Part model, mm, in its own coordinate system. Round coordinates to 2 decimals unless told otherwise and drop trailing zeros. Write each loop counter-clockwise with the first axis right and the second up, starting at its lowest first coordinate (ties: lowest second). Pieces come first, ordered by that corner, then holes. Notation, with made-up numbers: M 27.25,53.25 L 39.25,53.25 A18 ccw 39.25,87.25 Z; hole C 37,12.5 d3. An arc over 180 degrees is marked long. Use a Markdown table: item, result. Add a question column.
1) Drop flat-ended pins along their axis: P1, Ø10, axis at y = -9, z = 11, coming from the -X side; P2, Ø6, axis at y = -4.5, z = -7.5, coming from the +X side; P3, Ø10, axis at x = 7, y = -4, coming from the -Z side. Give the stop position or say it passes through.
2) Slice it at C-C on z = -9. Write the cut outline in (x, y).
3) Wall check: probe 1 along X at (y, z) = (-14.5, 0); probe 2 along Z at (x, y) = (9, -10.5); probe 3 along X at (y, z) = (-6, -4.5). Give the ranges that are in metal, low to high.
4) Slice it at B-B on z = -3. Write the cut outline in (x, y).
5) Slice it at A-A on x = 0. Write the cut outline in (y, z), plus the area to 3 significant figures.
6) Two-plate mould, pull along X, no slides. Class faces 1 (the face through (12.626, -10.018, 12.518)), 2 (the face through (-12.518, -10.018, 12.626)), 3 (the face through (-5.299, -10.018, -12.926)), 4 (the face through (-5.056, -10.018, 16.036)): released by +X, released by -X, zero draft, split by the parting line, or undercut.
7) Slice it at D-D on y = -3.75. Give the number of separate pieces and of enclosed holes in the cut face, plus the area to 3 significant figures.
```python
from build123d import *

# Parameters (mm, degrees)
SKETCH1_W           = 5.08
SKETCH1_H           = 0.3048
CUT_EXTRUDE1_DEPTH  = 33.328922036
CIRPATTERN1_COUNT   = 8
BOSS_EXTRUDE1_START = -20.32
BOSS_EXTRUDE1_DEPTH = 20.32
SKETCH8_R           = 1.524
CUT_EXTRUDE2_DEPTH  = 33.328922036


with BuildPart() as part:
    # Sketch1 → Revolve1 (revolve)
    with BuildSketch(Plane.YZ):
        with Locations((-2.54, 14.4526)):
            Rectangle(SKETCH1_W, SKETCH1_H)
        Polygon((0, 14.3002), (0, 7.9502), (-20.32, 7.9502), (-20.32, 17.78), (0, 17.78), (0, 14.605), (-5.08, 14.605), (-5.08, 14.3002), align=None)
    revolve(axis=Axis((0, 0, 0), (0, -1, 0)))

    # Sketch2 → Cut-Extrude1 (cut, through all)
    with BuildSketch(Plane(origin=(0, 0, 0), x_dir=(-1, 0, 0), z_dir=(0, 1, 0))):
        with BuildLine():
            ThreePointArc((15.771052614, 8.209890343), (16.426578088, 6.804111427), (16.957087384, 5.346549115))
            Line((16.957087384, 5.346549115), (15.140256593, 4.773704567))
            ThreePointArc((15.140256593, 4.773704567), (15.498699113, 3.435978871), (15.739187174, 2.072103301))
            Line((15.739187174, 2.072103301), (13.850484713, 1.823450905))
            ThreePointArc((13.850484713, 1.823450905), (12.906597069, 5.34608755), (11.083146164, 8.504397163))
            Line((11.083146164, 8.504397163), (12.594484277, 9.664087686))
            ThreePointArc((12.594484277, 9.664087686), (13.388839202, 8.529631283), (14.081296977, 7.330259235))
            Line((14.081296977, 7.330259235), (15.771052614, 8.209890343))
        make_face()
    cut_extrude1 = extrude(amount=-CUT_EXTRUDE1_DEPTH, mode=Mode.SUBTRACT)

    # CirPattern1: Cut-Extrude1 ×8 about axis
    cirpattern1_axis = Axis((0, 0, 0), (0, 1, 0))
    for i in range(1, CIRPATTERN1_COUNT):
        add(cut_extrude1.rotate(cirpattern1_axis, i * 360 / CIRPATTERN1_COUNT), mode=Mode.SUBTRACT)

    # Sketch5 → Boss-Extrude1 (add)
    with BuildSketch(Plane(origin=(0, 0, 0), x_dir=(1, 0, 0), z_dir=(0, 1, 0)).offset(BOSS_EXTRUDE1_START)):
        with BuildLine():
            Line((-7.5692, -2.431643765), (-7.5692, 2.431643765))
            ThreePointArc((-7.5692, 2.431643765), (-7.9502, 0), (-7.5692, -2.431643765))
        make_face()
    extrude(amount=BOSS_EXTRUDE1_DEPTH)

    # Sketch8 → Cut-Extrude2 (cut, through all)
    with BuildSketch(Plane(origin=(0, 0, 0), x_dir=(-1, 0, 0), z_dir=(0, 1, 0))):
        with Locations(Location((-10.95375, 0, 0), (0, 0, 90))):
            Circle(SKETCH8_R)
        with Locations(Location((10.95375, 0, 0), (0, 0, 90))):
            Circle(SKETCH8_R)
    extrude(amount=-CUT_EXTRUDE2_DEPTH, mode=Mode.SUBTRACT)


solid = part.part
```
Entries:
| question | item | result |
|---|---|---|
| 1 | P1 | stops at x = -15.77 |
| 1 | P2 | stops at x = 17.2 |
| 1 | P3 | stops at z = -17.67 |
| 2 | outline | M -15.33,-20.32 L -13.08,-20.32 L -13.08,0 L -15.33,0 Z; M -11.73,-20.32 L 11.73,-20.32 L 11.73,0 L -11.73,0 Z; M 13.08,-20.32 L 15.33,-20.32 L 15.33,0 L 13.08,0 Z |
| 3 | probe 1 | x = -17.78 to -12.48, -9.43 to -7.57, 7.95 to 9.43, 12.48 to 17.78 |
| 3 | probe 2 | z = -15.33 to -13.08, -11.73 to 11.73, 13.08 to 15.33 |
| 3 | probe 3 | x = -17.2 to -15.22, -13.23 to -6.55, 6.55 to 13.23, 15.22 to 17.2 |
| 4 | outline | M -17.53,-20.32 L -15.59,-20.32 L -15.59,0 L -17.53,0 Z; M -13.64,-20.32 L -7.36,-20.32 L -7.36,0 L -13.64,0 Z; M 7.36,-20.32 L 13.64,-20.32 L 13.64,0 L 7.36,0 Z; M 15.59,-20.32 L 17.53,-20.32 L 17.53,0 L 15.59,0 Z |
| 5 | outline | M -20.32,-17.78 L 0,-17.78 L 0,-7.95 L -20.32,-7.95 Z; M -20.32,7.95 L 0,7.95 L 0,17.78 L -20.32,17.78 Z |
| 5 | area | 399 mm^2 |
| 6 | face 1 | released by +X |
| 6 | face 2 | released by -X |
| 6 | face 3 | undercut |
| 6 | face 4 | undercut |
| 7 | separate pieces | 1 |
| 7 | enclosed holes | 3 |
| 7 | area | 617 mm^2 |
